Design review of the part built by this model. Coordinates are the model's own, in mm. Face numbers are marked on the shaded views. A direction names the side the tool comes from. Coordinates: 2 decimals unless noted, no trailing zeros. Loops run counter-clockwise (first coordinate to the right, second up) from the corner with the lowest first, then second, coordinate; pieces in that order, holes last. Notation, with made-up numbers: M -34.5,-15 L -19.5,-15 A21 ccw -19.5,20 Z; hole C 86,20 d11. An arc over 180 degrees is marked long. Answer as a JSON object with one key per item and string values. Group by question number.
1. Consider section B-B (y = -1.75). State the section outline as (x, z) points.
2. Insertion check: pin 1 (1.6 mm diameter, centred on y = -1.5, z = 7, fed in from -X); pin 2 (1.2 mm diameter, centred on x = 0.5, z = 8.5, fed in from +Y); pin 3 (0.8 mm diameter, centred on y = -1.5, z = 7.5, fed in from +X). Each pin has a flat end and moves straight along its axis. Give the tip position at first contact, or say it passes through.
3. To check wall thickness, follow probe 1 along X at (y, z) = (-2, 7); probe 2 along Y at (x, z) = (1.75, 8); probe 3 along Y at (x, z) = (-2.5, 5). State the ranges of each line that lie inside material, in increasing order.
4. Consider section D-D (x = -2.5). State the section outline as (y, z) points, then the cut area to 3 significant figures.
5. Consider section C-C (z = 0). State the section outline as (x, y) points, then the cut area to 3 significant figures.
6. Consider section A-A (x = 0). State the section outline as (y, z) points.
7. Machinability: for the marked faces 1 and 2, which of the approach directions +Z, -Z, +X, -X, +Y, -Y give a long, thin tool a straight path to every point of the face, cutting with its end or side? Answer none if there is none.
8. Draft analysis for pull direction Z (two halves, no side actions). For the marked faces 3 and 4, state which applies: +Z half, -Z half, draft (parallel to the pull), parting line (faces both ways), or undercut.
from build123d import *

# Parameters (mm, degrees)
BOSS_EXTRUDE1_DEPTH = 1.5


with BuildPart() as part:
    # Sketch1 → Revolve1 (revolve)
    with BuildSketch(Plane(origin=(0, 0, 0), x_dir=(0, 0, -1), z_dir=(1, 0, 0))):
        with BuildLine():
            Line((4.3, 0), (6, 0))
            Line((6, 0), (6, -2.5))
            Line((6, -2.5), (0, -2.5))
            Line((0, -2.5), (0, 4.3))
            ThreePointArc((0, 4.3), (3.040559159, 3.040559159), (4.3, 0))
        make_face()
    revolve(axis=Axis((0, -2.5, 0), (0, 1, 0)))

    # Sketch2 → Boss-Extrude1 (add)
    with BuildSketch(Plane.XZ.offset(2.5)):
        with BuildLine():
            Line((0, 10), (-2, 10))
            Line((-2, 10), (-2, 5.656854249))
            ThreePointArc((-2, 5.656854249), (0, 6), (2, 5.656854249))
            Line((2, 5.656854249), (2, 10))
            Line((2, 10), (0, 10))
        make_face()
        with BuildLine():
            Line((0, -10), (-2, -10))
            Line((-2, -10), (-2, -5.656854249))
            ThreePointArc((-2, -5.656854249), (0, -6), (2, -5.656854249))
            Line((2, -5.656854249), (2, -10))
            Line((2, -10), (0, -10))
        make_face()
    extrude(amount=-BOSS_EXTRUDE1_DEPTH)


solid = part.part
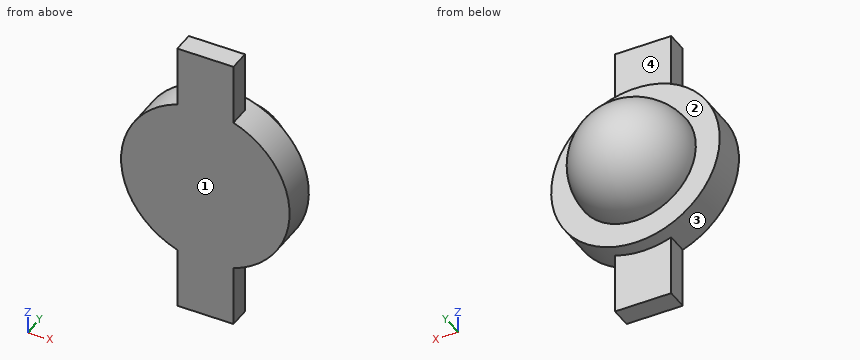
Findings below:
{
 "1": {"outline": "M -2,-10 L 2,-10 L 2,-5.66 A6 ccw 2,5.66 L 2,10 L -2,10 L -2,5.66 A6 ccw -2,-5.66 Z"},
 "2": {"pin 1": "stops at x = -2", "pin 2": "stops at y = -1", "pin 3": "stops at x = 2"},
 "3": {"probe 1": "x = -2 to 2", "probe 2": "y = -2.5 to -1", "probe 3": "y = -2.5 to 0"},
 "4": {"outline": "M -2.5,-5.45 L 0,-5.45 L 0,-3.5 A3.5 ccw 0,3.5 L 0,5.45 L -2.5,5.45 Z", "area": "46.5 mm^2"},
 "5": {"outline": "M -6,-2.5 L 6,-2.5 L 6,0 L 4.3,0 A4.3 ccw -4.3,0 L -6,0 Z", "area": "59.0 mm^2"},
 "6": {"outline": "M -2.5,-10 L -1,-10 L -1,-6 L 0,-6 L 0,-4.3 A4.3 ccw 0,4.3 L 0,6 L -1,6 L -1,10 L -2.5,10 Z"},
 "7": {"face 1": "+Z, -Z, +X, -X, -Y", "face 2": "+Y"},
 "8": {"face 3": "parting line", "face 4": "draft"}
}
